Solid Edge part; units mm, degrees
sketch "Sketch1" plane through (0, 0, 0) normal (1, 0, 0) x (0, 1, 0)
  line L0 (3, 0) -> (-1.5, 0)
  line L1 (-1.5, 0) -> (-1.5, 2)
  arc A0 (-1.5, 2) -> (-1, 2.5) centre (-1, 2) cw
  line L2 (-1, 2.5) -> (0, 2.5)
  line L3 (0, 2.5) -> (0, 1.25)
  line L4 (0, 1.25) -> (3, 1.25)
  line L5 (3, 1.25) -> (3, 0)
revolve "RevolvedProtrusion1" add sketch "Sketch1" angle 360 about axis through (0, 38.2678, 0) along (0, -1, 0)
sketch "Sketch2" plane through (0, 0, 0) normal (1, 0, 0) x (0, 1, 0)
  line L0 (-1, -0.4) -> (-1.5, -0.4)
  line L1 (-1.5, -0.4) -> (-1.5, 0.4)
  line L2 (-1.5, 0.4) -> (-1, 0.4)
  line L3 (-1, 0.4) -> (-1, -0.4)
extrude "Cutout1" cut sketch "Sketch2" against normal up to next and the other way up to next
Can you work these out from the model? Positions are in its coordinate system, mm. A direction names the side the tool comes from. Give positions to 0.01 mm unless a question says otherwise; leave off trailing zeros. Order: outer loops, then holes, each group sorted by start corner. A loop starts at its lowest first (then second) coordinate and runs counter-clockwise, first axis right, second up. Notation, with made-up numbers: M 48,-11 L 105,-11 A25 cw 105,20 Z; hole C -10.75,21 d11. An arc over 180 degrees is marked long. Use a Markdown table: item, result. Add a question column.
Item 1: Suppose I cut it at A-A (x = 0). List the corners of the cut face in (y, z) for me, then the cut area to 3 significant figures.
Item 2: Suppose I cut it at B-B (z = 0). List the corners of the cut face in (x, y) for me.
Item 3: If I drill on L1, parallel to Y at x = 1.85, z = -0.1; L2, parallel to Z at x = 0.05, y = 2.75; L3, parallel to Y at x = 0.6, z = 1.55, over which ranges is the centre line in solid material (lowest first)? Write a range as [from, to].
Item 4: Suppose I cut it at C-C (y = 1.5). List the corners of the cut face in (x, z) for me, then the cut area to 3 significant figures.
Item 5: For faces 1 (the flat face through (0, 3, 0)), 2 (the cylindrical face through (-1.22, 1.52, -0.27)), which set-ups out of +Z, -Z, +X, -X, +Y, -Y let a thin tool reach every point of the face, with its end or its side?
Item 6: Will these pins go through, and if not, where does the flat tip stop? pin 1 (0.6 mm diameter, centred on x = 0.5, y = -1.5, fed in from -Z); pin 2 (0.6 mm diameter, centred on x = 0.5, z = 0, fed in from -Y).
Item 7: Suppose I cut it at D-D (y = -0.35). List the corners of the cut face in (x, z) for me.
Answer sheet:
| question | item | result |
|---|---|---|
| 1 | outline | M -1.5,-2 A0.5 ccw -1,-2.5 L 0,-2.5 L 0,-1.25 L 3,-1.25 L 3,1.25 L 0,1.25 L 0,2.5 L -1,2.5 A0.5 ccw -1.5,2 L -1.5,0.4 L -1,0.4 L -1,-0.4 L -1.5,-0.4 Z |
| 1 | area | 14.5 mm² |
| 2 | outline | M -2.5,-1 L 2.5,-1 L 2.5,0 L 1.25,0 L 1.25,3 L -1.25,3 L -1.25,0 L -2.5,0 Z |
| 3 | L1 | y = [-1, 0] |
| 3 | L2 | z = [-1.25, 1.25] |
| 3 | L3 | y = [-1.5, 0] |
| 4 | outline | C 0,0 d2.5 |
| 4 | area | 4.91 mm² |
| 5 | face 1 | +Z, -Z, +X, -X, +Y |
| 5 | face 2 | +Y |
| 6 | pin 1 | stops at z = -2.42 |
| 6 | pin 2 | stops at y = -1 |
| 7 | outline | C 0,0 d5 |
